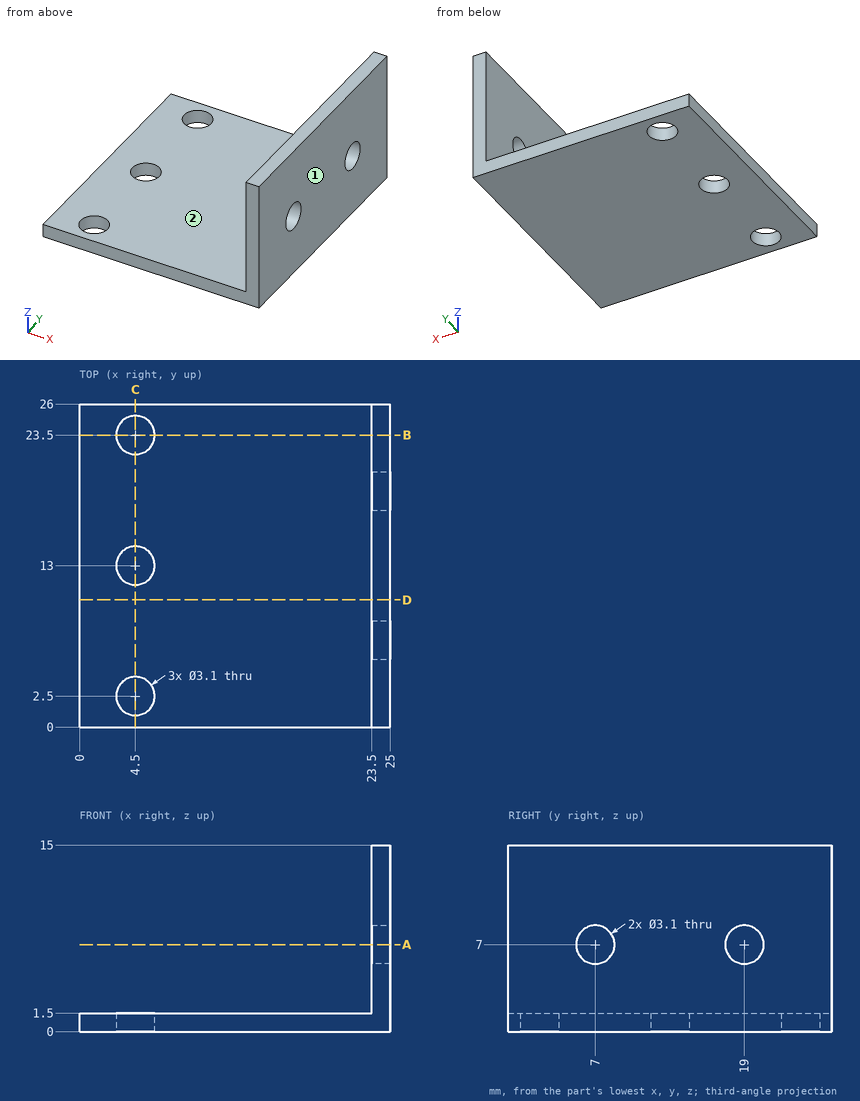
Drawing for the job (mm, zero at the part's lowest x, y, z). A direction names the side the tool comes from. Give positions to 0.01 mm unless a question says otherwise; leave off trailing zeros. Write each loop counter-clockwise with the first axis right and the second up, starting at its lowest first coordinate (ties: lowest second). Pieces come first, ordered by that corner, then holes. Notation, with made-up numbers: (43.5, -1.75) -> (101.5, -1.75) arc R11 cw to (101.5, 19.25) -> close; hole circle Ø3 at (-6.5, 14). An arc over 180 degrees is marked (long way). Put each result on its own line as item: value. Start each with the question number.
Item 1: Cut at B-B (y = 23.5). List the corners of the cut face in (x, z), then the cut area to 3 significant figures.
Item 2: Cut at D-D (y = 10.25). List the corners of the cut face in (x, z), then the cut area to 4 significant figures.
Item 3: Wall check: L1, parallel to Y at x = 24.3, z = 7; L2, parallel to Y at x = 4.5, z = 0.45; L3, parallel to X at y = 18, z = 2.75. Give the ranges that are in metal, low to high. Write a range as [from, to].
Item 4: Pin check, flat tips, straight feed: pin 1 Ø10 at (x, y) = (10, 9.5) entering from +Z; pin 2 Ø3 at (x, z) = (20.5, 11) entering from +Y; pin 3 Ø5 at (y, z) = (19, 7) entering from -X. Stop position of each tip, or through.
Item 5: Cut at A-A (z = 7). List the corners of the cut face in (x, y).
Item 6: Cut at C-C (x = 4.5). List the corners of the cut face in (y, z).
Item 7: Which spindle directions (+Z, -Z, +X, -X, +Y, -Y) get a long thin tool onto all of the face, cutting with end or side? Do the marked faces 1 and 2. Say none if no direction does.
Answer list:
1. outline: (0, 0) -> (2.95, 0) -> (2.95, 1.5) -> (0, 1.5) -> close; (6.05, 0) -> (25, 0) -> (25, 15) -> (23.5, 15) -> (23.5, 1.5) -> (6.05, 1.5) -> close
1. area: 53.1 mm2
2. outline: (0, 0) -> (25, 0) -> (25, 15) -> (23.5, 15) -> (23.5, 1.5) -> (0, 1.5) -> close
2. area: 57.75 mm2
3. L1: y = [0, 5.45], [8.55, 17.45], [20.55, 26]
3. L2: y = [0, 0.95], [4.05, 11.45], [14.55, 21.95], [25.05, 26]
3. L3: x = [23.5, 25]
4. pin 1: stops at z = 1.5
4. pin 2: passes through
4. pin 3: stops at x = 23.5
5. outline: (23.5, 0) -> (25, 0) -> (25, 5.45) -> (23.5, 5.45) -> close; (23.5, 8.55) -> (25, 8.55) -> (25, 17.45) -> (23.5, 17.45) -> close; (23.5, 20.55) -> (25, 20.55) -> (25, 26) -> (23.5, 26) -> close
6. outline: (0, 0) -> (0.95, 0) -> (0.95, 1.5) -> (0, 1.5) -> close; (4.05, 0) -> (11.45, 0) -> (11.45, 1.5) -> (4.05, 1.5) -> close; (14.55, 0) -> (21.95, 0) -> (21.95, 1.5) -> (14.55, 1.5) -> close; (25.05, 0) -> (26, 0) -> (26, 1.5) -> (25.05, 1.5) -> close
7. face 1: +Z, -Z, +X, +Y, -Y
7. face 2: +Z, -X, +Y, -Y
